Verification items for the finished model (mm, model axes). Face numbers are marked on the shaded views. A direction names the side the tool comes from. Give positions to 0.01 mm unless a question says otherwise; leave off trailing zeros. Loops run counter-clockwise (first coordinate to the right, second up) from the corner with the lowest first, then second, coordinate; pieces in that order, holes last. Notation, with made-up numbers: (-30, -17) - (1, -17) arc R20 ccw to (1, 3) - close; hole circle Ø1 at (56.25, 81). An arc over 180 degrees is marked (long way). Answer in a Markdown table with one row per item.
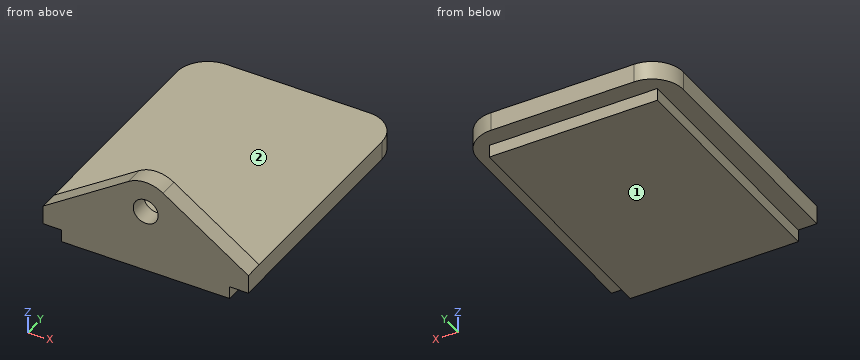
```python
from build123d import *

# Parameters (mm, degrees)
EXTRUDE_1_DEPTH = 3
SKETCH_2_R      = 2
EXTRUDE_2_DEPTH = 3
SKETCH_3_W      = 27
SKETCH_3_H      = 39
EXTRUDE_3_DEPTH = 2


with BuildPart() as part:
    # 草图1 → 凸台-拉伸1 (new body)
    with BuildSketch(Plane.XY):
        with BuildLine():
            Line((11.5, 23.5), (-11.5, 23.5))
            ThreePointArc((-11.5, 23.5), (-15.035533906, 22.035533906), (-16.5, 18.5))
            Line((-16.5, 18.5), (-16.5, -18.5))
            Line((-16.5, -18.5), (16.5, -18.5))
            Line((16.5, -18.5), (16.5, 18.5))
            ThreePointArc((16.5, 18.5), (15.035533906, 22.035533906), (11.5, 23.5))
        make_face()
    extrude(amount=EXTRUDE_1_DEPTH)

    # 草图2 → 凸台-拉伸2 (add)
    with BuildSketch(Plane.XZ.offset(18.5)):
        with BuildLine():
            ThreePointArc((-1.2e-08, 3), (-4.785122024, 6.549963029), (-2.775441548, 12.158957107))
            Line((-2.775441548, 12.158957107), (-16.5, 3))
            Line((-16.5, 3), (-1.2e-08, 3))
        make_face()
        with BuildLine():
            Line((16.5, 3), (2.775441548, 12.158957107))
            ThreePointArc((2.775441548, 12.158957107), (4.40892321, 10.358261252), (5, 8))
            ThreePointArc((5, 8), (3.535533902, 4.46446609), (-1.2e-08, 3))
            Line((-1.2e-08, 3), (16.5, 3))
        make_face()
        with BuildLine():
            ThreePointArc((2.775441548, 12.158957107), (0, 13), (-2.775441548, 12.158957107))
            ThreePointArc((-2.775441548, 12.158957107), (-4.785122024, 6.549963029), (-1.2e-08, 3))
            ThreePointArc((-1.2e-08, 3), (3.535533902, 4.46446609), (5, 8))
            ThreePointArc((5, 8), (4.40892321, 10.358261252), (2.775441548, 12.158957107))
        make_face()
        with Locations(Location((0, 8, 0), (0, 0, 270))):
            Circle(SKETCH_2_R, mode=Mode.SUBTRACT)
    extrude(amount=-EXTRUDE_2_DEPTH)

    # 草图3 → 凸台-拉伸3 (add)
    with BuildSketch(Plane(origin=(0, 0, 0), x_dir=(-1, 0, 0), z_dir=(0, 0, -1))):
        with Locations((0, 1)):
            Rectangle(SKETCH_3_W, SKETCH_3_H)
    extrude(amount=EXTRUDE_3_DEPTH)


solid = part.part
```
Q1. Go/stop test with flat-tipped pins: P1, Ø10, axis at x = -5.5, y = -0.5, coming from the +Z side; P2, Ø5, axis at x = 4.5, z = 6.5, coming from the +Y side; P3, Ø1, axis at y = 10.5, z = -1.5, coming from the -X side; P4, Ø2.5, axis at x = 0, z = 8, coming from the -Y side. Record where each tip stops, or that it passes through.
Completed:
| item | result |
|---|---|
| P1 | z = 3 |
| P2 | y = -15.5 |
| P3 | x = -13.5 |
| P4 | through |
Q2. Tool access check on the marked faces 1 and 2. Record the directions out of +Z, -Z, +X, -X, +Y, -Y that give a thin tool (end or side, any length) a straight path to the whole face; none if there is none.
Completed:
| item | result |
|---|---|
| face 1 | -Z, +X, -X, +Y, -Y |
| face 2 | +Z, +X, -X, +Y |
Q3. Sectioned sample at A-A (x = 1). Record the cut outline in (y, z), and give its area (3 significant figures).
Completed:
| item | result |
|---|---|
| outline | (-18.5, -2) - (20.5, -2) - (20.5, 0) - (23.5, 0) - (23.5, 3) - (-15.5, 3) - (-15.5, 6.27) - (-18.5, 6.27) - close; (-18.5, 9.73) - (-15.5, 9.73) - (-15.5, 12.9) - (-18.5, 12.9) - close |
| area | 223 mm^2 |
Q4. Sectioned sample at D-D (x = 10.5). Record the cut outline in (y, z), and give its area (3 significant figures).
Completed:
| item | result |
|---|---|
| outline | (-18.5, -2) - (20.5, -2) - (20.5, 0) - (23.5, 0) - (23.5, 3) - (-15.5, 3) - (-15.5, 7) - (-18.5, 7) - close |
| area | 216 mm^2 |
Q5. Sectioned sample at B-B (y = -8). Record the cut outline in (x, z).
Completed:
| item | result |
|---|---|
| outline | (-16.5, 0) - (-13.5, 0) - (-13.5, -2) - (13.5, -2) - (13.5, 0) - (16.5, 0) - (16.5, 3) - (-16.5, 3) - close |
Q6. Thickness scan on line 1 (Z direction, x = 2.5, y = 14); line 2 (Y direction, x = -8, z = 4.5); line 3 (X direction, y = -17.35, z = 8). Record the ranges inside material, lowest first.
Completed:
| item | result |
|---|---|
| line 1 | -2 to 3 |
| line 2 | -18.5 to -15.5 |
| line 3 | -9.01 to -2, 2 to 9.01 |
Q7. Sectioned sample at C-C (z = 8.75). Record the cut outline in (x, y).
Completed:
| item | result |
|---|---|
| outline | (-7.88, -18.5) - (-1.85, -18.5) - (-1.85, -15.5) - (-7.88, -15.5) - close; (1.85, -18.5) - (7.88, -18.5) - (7.88, -15.5) - (1.85, -15.5) - close |
